Can you work these out from the model? Positions are in its coordinate system, mm. A direction names the side the tool comes from. Give positions to 0.01 mm unless a question says otherwise; leave off trailing zeros. Loops run counter-clockwise (first coordinate to the right, second up) from the corner with the lowest first, then second, coordinate; pieces in that order, holes last. Notation, with made-up numbers: M 39.5,-18.5 L 74.5,-18.5 A14 cw 74.5,-7.5 Z; hole C 11.5,55 d3. An arc over 180 degrees is marked long. Use CSV: the item, a comma, the result in double quotes.
from build123d import *

# Parameters (mm, degrees)
SKETCH1_W            = 34
SKETCH1_H            = 38
BOSS_EXTRUDE1_DEPTH  = 12
SKETCH_1_R           = 12.5
EXTRUDE_1_DEPTH      = 6
SKETCH_2_R           = 5
CUT_EXTRUDE_1_DEPTH  = 100
SKETCH2_R            = 3
CUT_EXTRUDE1_DEPTH   = 5
LPATTERN1_COUNT      = 2
LPATTERN1_PITCH      = 24
LPATTERN1_COUNT_DIR2 = 2
LPATTERN1_PITCH_DIR2 = 28


with BuildPart() as part:
    # Sketch1 → Boss-Extrude1 (new body)
    with BuildSketch(Plane.XY):
        with Locations((-1.444444444, -6.888888889)):
            Rectangle(SKETCH1_W, SKETCH1_H)
    extrude(amount=BOSS_EXTRUDE1_DEPTH)

    # Эскиз1 → Бобышка-Вытянуть1 (add)
    with BuildSketch(Plane.XY.offset(12)):
        with Locations((-1.444444444, -6.888888889)):
            Circle(SKETCH_1_R)
    extrude(amount=EXTRUDE_1_DEPTH)

    # Эскиз2 → Вырез-Вытянуть1 (cut)
    with BuildSketch(Plane.XY.offset(18)):
        with Locations((-1.444444444, -6.888888889)):
            Circle(SKETCH_2_R)
    extrude(amount=-CUT_EXTRUDE_1_DEPTH, mode=Mode.SUBTRACT)

    # Sketch2 → Cut-Extrude1 (cut)
    with BuildSketch(Plane.XY.offset(12)):
        with Locations((-13.444444444, 7.111111111)):
            Circle(SKETCH2_R)
    cut_extrude1 = extrude(amount=-CUT_EXTRUDE1_DEPTH, mode=Mode.SUBTRACT)

    # LPattern1: Cut-Extrude1 2 × 2
    with Locations(*[(i * LPATTERN1_PITCH, -j * LPATTERN1_PITCH_DIR2, 0) for i in range(LPATTERN1_COUNT) for j in range(LPATTERN1_COUNT_DIR2) if (i, j) != (0, 0)]):
        add(cut_extrude1, mode=Mode.SUBTRACT)


solid = part.part
Q1. I'm going to push flat-ended pins straight in: P1, Ø3.5, axis at x = 10.56, y = 7.11, coming from the +Z side; P2, Ø7, axis at x = -13.44, y = -20.89, coming from the +Z side. Where does each tip first touch, or does it pass through?
Model answer:
P1,"z = 7"
P2,"z = 12"
Q2. I want a section at D-D, the plane x = -8. Please give me the cut outline in (y, z).
Model answer:
outline,"M -25.89,0 L 12.11,0 L 12.11,12 L 3.75,12 L 3.75,18 L -17.53,18 L -17.53,12 L -25.89,12 Z"
Q3. If we mould it in two halves opening along Y, with no side actions, what happens to faces 3 (the flat face through (-2, 12.111, 6)), 4 (the flat face through (-5, -2, 0)), 5 (the cylindrical face through (-11.83, 9.64, 9.54)), 6 (the flat face through (-2, -25.889, 6))? For each: released by +Y, released by -Y, zero draft, split by the parting line, or undercut.
Model answer:
face 3,"released by +Y"
face 4,"zero draft"
face 5,"undercut"
face 6,"released by -Y"
Q4. For faces 1 (the flat face through (-13, -21, 7)), 2 (the flat face through (-18.444, -7, 6)), which set-ups out of +Z, -Z, +X, -X, +Y, -Y let a thin tool reach every point of the face, with its end or its side?
Model answer:
face 1,"+Z"
face 2,"+Z, -Z, -X, +Y, -Y"
Q5. I want a section at C-C, the plane y = -22. Please give me the cut outline in (x, z), then the cut area to 3 significant figures.
Model answer:
outline,"M -18.44,0 L 15.56,0 L 15.56,12 L 13.34,12 L 13.34,7 L 7.77,7 L 7.77,12 L -10.66,12 L -10.66,7 L -16.23,7 L -16.23,12 L -18.44,12 Z"
area,"352 mm2"
Q6. Please list where these lines run through material, in increasing order: L1, parallel to Y at x = -13.5, z = 9.75; L2, parallel to Y at x = 12.5, z = 10; L3, parallel to Z at x = 10, y = -12. Write a range as from..to.
Model answer:
L1,"-25.89..-23.89, -17.89..4.11, 10.11..12.11"
L2,"-25.89..-23.17, -18.6..4.83, 9.4..12.11"
L3,"0..12"
Q7. I want a section at A-A, the plane x = 2.5. Please give me the cut outline in (y, z), then the cut area to 3 significant figures.
Model answer:
outline,"M -25.89,0 L -9.96,0 L -9.96,18 L -18.75,18 L -18.75,12 L -25.89,12 Z; M -3.82,0 L 12.11,0 L 12.11,12 L 4.97,12 L 4.97,18 L -3.82,18 Z"
area,"488 mm2"
Q8. I want a section at B-B, the plane z = 9.75. Please give me the cut outline in (x, y).
Model answer:
outline,"M -18.44,-25.89 L 15.56,-25.89 L 15.56,12.11 L -18.44,12.11 Z; hole C -13.44,-20.89 d6; hole C -13.44,7.11 d6; hole C -1.44,-6.89 d10; hole C 10.56,-20.89 d6; hole C 10.56,7.11 d6"
